Check sheet for the modelled part. Datum: model origin and axes. Units: mm. Face numbers are marked on the shaded views. Coordinates: 2 decimals unless noted, no trailing zeros. Write each loop counter-clockwise with the first axis right and the second up, starting at its lowest first coordinate (ties: lowest second). Pieces come first, ordered by that corner, then holes. Notation, with made-up numbers: (-27, -8) - (-5, -8) arc R11 ccw to (-5, -1) - close; hole circle Ø10 at (70.5, 40.5). An arc over 180 degrees is marked (long way). Use one line per item in the form item = value. Start each with the question number.
1. Scan lines: line 1 along Z through (x, y) = (-6, -17.5) (3 decimals); line 2 along Z through (x, y) = (3, -10) (3 decimals); line 3 along Y through (x, z) = (1.5, 10). Record each from-to range of solid material in increasing order.
2. Cross-section at B-B on y = -30. Record the boundary of the cut face in (x, z) (3 decimals), then the cut area to 3 significant figures.
3. Cross-section at A-A on x = 4.5. Record the boundary of the cut face in (y, z) (3 decimals).
4. Draft check along X on the marked faces 1 and 2. Enter one of: +X half, -X half, draft (parallel to the pull), parting line (faces both ways), or undercut.
```python
from build123d import *

# Parameters (mm, degrees)
SKETCH1_W           = 412.75
SKETCH1_H           = 101.6
BOSS_EXTRUDE1_DEPTH = 9.525
CUT_EXTRUDE1_REACH  = 21.05
SKETCH2_R           = 15.875
FILLET1_R           = 31.75


with BuildPart() as part:
    # Sketch1 → Boss-Extrude1 (new body, symmetric)
    with BuildSketch(Plane(origin=(0, 0, 0), x_dir=(0, 0, -1), z_dir=(1, 0, 0))):
        Rectangle(SKETCH1_W, SKETCH1_H)
    extrude(amount=BOSS_EXTRUDE1_DEPTH, both=True)

    # Sketch2 → Cut-Extrude1 (cut, up to next)
    with BuildSketch(Plane(origin=(9.525, 0, 0), x_dir=(0, 0, -1), z_dir=(1, 0, 0)), mode=Mode.PRIVATE) as cut_extrude1_sk1:
        with Locations((-174.625, -19.05)):
            Circle(SKETCH2_R)
    cut_extrude1_tool1 = extrude(cut_extrude1_sk1.sketch, amount=-CUT_EXTRUDE1_REACH, mode=Mode.PRIVATE) & part.part
    add(cut_extrude1_tool1.solids().sort_by_distance((9.525, -19.05, 174.625))[0], mode=Mode.SUBTRACT)
    # Sketch2 → Cut-Extrude1 (cut, up to next)
    with BuildSketch(Plane(origin=(9.525, 0, 0), x_dir=(0, 0, -1), z_dir=(1, 0, 0)), mode=Mode.PRIVATE) as cut_extrude1_sk2:
        with Locations((3.175, -19.05)):
            Circle(SKETCH2_R)
    cut_extrude1_tool2 = extrude(cut_extrude1_sk2.sketch, amount=-CUT_EXTRUDE1_REACH, mode=Mode.PRIVATE) & part.part
    add(cut_extrude1_tool2.solids().sort_by_distance((9.525, -19.05, -3.175))[0], mode=Mode.SUBTRACT)

    # Fillet1
    fillet1_edges = [part.edges().sort_by_distance(p)[0] for p in [
        (0, -50.8, 206.375),
    ]]
    fillet(fillet1_edges, radius=FILLET1_R)


solid = part.part
```
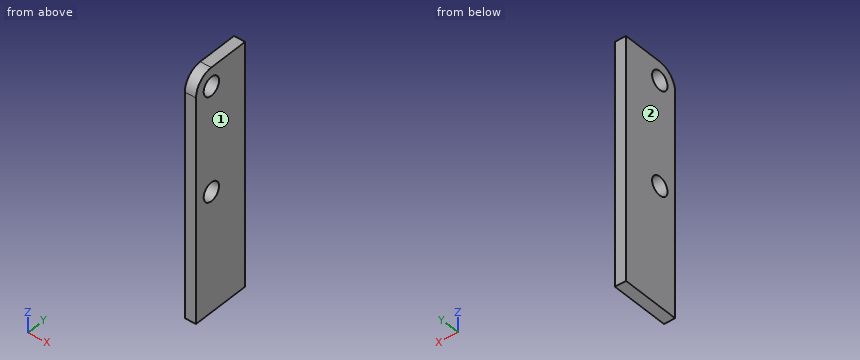
Final values:
q1.line_1 = -206.375 to -18.974, 12.624 to 158.826, 190.424 to 206.375
q1.line_2 = -206.375 to -16.218, 9.868 to 161.582, 187.668 to 206.375
q1.line_3 = -50.8 to -27.91, -10.19 to 50.8
q2.outline = (-9.525, -206.375) - (9.525, -206.375) - (9.525, -14.669) - (-9.525, -14.669) - close; (-9.525, 8.319) - (9.525, 8.319) - (9.525, 163.131) - (-9.525, 163.131) - close; (-9.525, 186.119) - (9.525, 186.119) - (9.525, 204.427) - (-9.525, 204.427) - close
q2.area = 6,950 mm²
q3.outline = (-50.8, -206.375) - (50.8, -206.375) - (50.8, 206.375) - (-19.05, 206.375) arc R31.75 ccw to (-50.8, 174.625) - close; hole circle Ø31.75 at (-19.05, -3.175); hole circle Ø31.75 at (-19.05, 174.625)
q4.face_1 = +X half
q4.face_2 = -X half
